CAD build for the part. Positions are in the model's coordinates, mm. A direction names the side the tool comes from. Coordinates: 2 decimals unless noted, no trailing zeros. Order: outer loops, then holes, each group sorted by start corner. A loop starts at its lowest first (then second) coordinate and runs counter-clockwise, first axis right, second up. Notation, with made-up numbers: M 87,45.25 L 129,45.25 A21 ccw 129,75.25 Z; hole C 43.5,-19 d4. An arc over 180 degrees is marked long. One line per item, written item: value.
from build123d import *


# Read off the part's stored shape, not the designer's step: Shell1
with BuildPart() as part:
    # Sketch3 → Revolve3 (revolve)
    with BuildSketch(Plane(origin=(0, 0, 0), x_dir=(0, 0, -1), z_dir=(1, 0, 0)), mode=Mode.PRIVATE) as revolve3_sk:
        with BuildLine():
            Line((40.933444221, 9.132480421), (48.707266624, 9.132480421))
            Line((48.707266624, 9.132480421), (50.458444221, 7.663067945))
            Line((50.458444221, 7.663067945), (50.458444221, 4.369980421))
            Line((50.458444221, 4.369980421), (-38.441555779, 4.369980421))
            ThreePointArc((-38.441555779, 4.369980421), (-35.186779885, 12.227704527), (-27.329055779, 15.482480421))
            Line((-27.329055779, 15.482480421), (24.901639323, 15.482480421))
            ThreePointArc((24.901639323, 15.482480421), (31.916856339, 14.14375452), (37.946094067, 10.315732937))
            ThreePointArc((37.946094067, 10.315732937), (39.32686809, 9.439066101), (40.933444221, 9.132480421))
        make_face()
    revolve(revolve3_sk.sketch.rotate(Axis((0, 4.369980421, 38.441555779), (0, 0, -1)), 180), axis=Axis((0, 4.369980421, 38.441555779), (0, 0, -1)))

    # Shell1 outline → Shell1 (revolve, cut)
    with BuildSketch(Plane.XZ.offset(-4.369980421)):
        with BuildLine():
            ThreePointArc((4.09465218, -36.206833435), (7.412270886, -30.981494071), (8.5725, -24.901639323))
            Line((8.5725, -24.901639323), (8.5725, 27.329055776))
            ThreePointArc((8.5725, 27.329055776), (6.061672883, 33.39072866), (0, 35.901555779))
            Line((0, 35.901555779), (0, -47.918444221))
            Line((0, -47.918444221), (2.108666073, -47.918444221))
            Line((2.108666073, -47.918444221), (2.2225, -47.782782229))
            Line((2.2225, -47.782782229), (2.2225, -40.933444221))
            ThreePointArc((2.2225, -40.933444221), (2.707582467, -38.391505822), (4.09465218, -36.206833435))
        make_face()
    revolve(axis=Axis((0, 4.369980421, 0), (0, 0, 1)), mode=Mode.SUBTRACT)


solid = part.part
Q1. Drill centre lines: line 1 along X through (y, z) = (-2.5, 12); line 2 along Z through (x, y) = (-3, 8.5); line 3 along X through (y, z) = (11.5, -16). Where is each one in solid material? Low to high.
Recorded:
line 1: x = -8.73 to -5.13, 5.13 to 8.73
line 2: z = -39.24 to -35.03, 34.22 to 37.2
line 3: x = -8.52 to -4.76, 4.76 to 8.52
Q2. Which spindle directions (+Z, -Z, +X, -X, +Y, -Y) get a long thin tool onto all of the face, cutting with end or side? Do faces 4 (the face through (4.609, 11.598, 1.579)), 5 (the face through (4.65, 5.4, -44.87)). Say none if no direction does.
Recorded:
face 4: none
face 5: -Z
Q3. Slice it at B-B (z = 3). List the corners of the cut face in (x, y) (1 decimal).
Recorded:
outline: C 0,4.4 d22.2; hole C 0,4.4 d17.1
Q4. Pin check, flat tips, straight feed: pin 1 Ø2 at (x, z) = (-8.5, -11) entering from -Y; pin 2 Ø1 at (x, z) = (2.5, -3) entering from +Y; pin 3 Ø4 at (x, y) = (1.5, 8.5) entering from -Z; pin 4 Ø1.5 at (y, z) = (2.5, -21.5) entering from +X. Stop position of each tip, or through.
Recorded:
pin 1: stops at y = -3.83
pin 2: stops at y = 15.3
pin 3: stops at z = -50.46
pin 4: stops at x = 11.06
Q5. Slice it at A-A (z = -45). List the corners of the cut face in (x, y) (1 decimal).
Recorded:
outline: C 0,4.4 d9.5; hole C 0,4.4 d4.4
Q6. Mould opens along Y. For faces 1 (the face through (-7.51, 12.56, 0.85)), 2 (the face through (0, 4, -47.918)), 3 (the face through (0, 4, -50.458)) say: released by +Y, released by -Y, zero draft, split by the parting line, or undercut.
Recorded:
face 1: split by the parting line
face 2: undercut
face 3: zero draft
